Build history of the part. All positions in model axes, mm. Face numbers are marked on the shaded views. A direction names the side the tool comes from. Round coordinates to 2 decimals unless told otherwise and drop trailing zeros. Loops run counter-clockwise (first coordinate to the right, second up) from the corner with the lowest first, then second, coordinate; pieces in that order, holes last. Notation, with made-up numbers: (86.25, -1) - (109.25, -1) arc R18 cw to (109.25, 28) - close; hole circle Ø3 at (-1, 58). An arc over 180 degrees is marked (long way). Put each result on its own line as item: value. Start each with the question number.
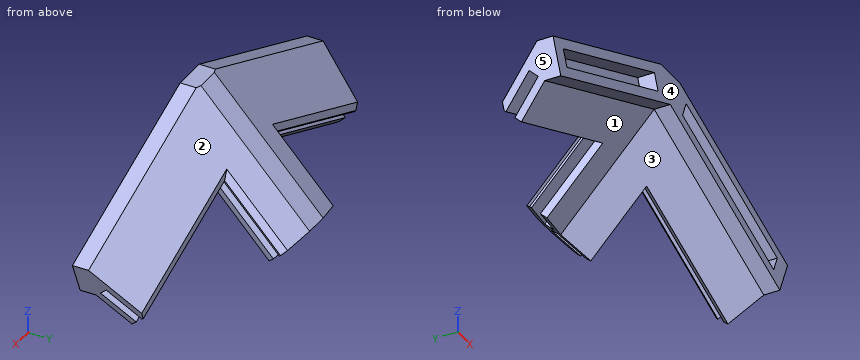
from build123d import *

# Parameters (mm, degrees)
SKETCH1_W                = 214.0895226738578
SKETCH1_H                = 271.0335668448457
BOSS_EXTRUDE1_DEPTH      = 10
SKETCH3_W                = 107.0447613369289
SKETCH3_H                = 271.0335668448457
CUT_EXTRUDE1_DEPTH       = 252.25359017903727
CUT_EXTRUDE2_DEPTH       = 249.55642867000518
BOSS_EXTRUDE3_DEPTH      = 40
CUT_EXTRUDE3_START       = -165.689856025
CUT_EXTRUDE3_DEPTH       = 205.862728092
CUT_EXTRUDE4_DEPTH       = 250.9605933606232
CUT_EXTRUDE5_DEPTH       = 250.96059336062322
BOSS_EXTRUDE5_DEPTH      = 45.000000000000014
CUT_EXTRUDE7_DEPTH       = 253.78419033582136
CUT_EXTRUDE9_DEPTH       = 253.78419033582136
CUT_EXTRUDE10_DEPTH      = 105
BOSS_EXTRUDE6_DEPTH      = 13.546139965279659
BOSS_EXTRUDE7_DEPTH      = 30
CUT_EXTRUDE12_DEPTH      = 30
CUT_EXTRUDE13_DEPTH      = 30
CUT_EXTRUDE14_DEPTH      = 30
CUT_EXTRUDE14_DEPTH_BACK = 101.66514829221025
BOSS_EXTRUDE8_DEPTH      = 5.2
CHAMFER1_START           = 223.359720619
CHAMFER1_OUTLINE_W       = 14
CHAMFER1_OUTLINE_H       = 9.000000000000002
CHAMFER1_DEPTH           = 3.640279381
CHAMFER3_START           = 159.35770891
CHAMFER3_OUTLINE_W       = 10
CHAMFER3_OUTLINE_H       = 51.999999999999986
CHAMFER3_DEPTH           = 1.64229109
CHAMFER4_SIZE            = 1.7


with BuildPart() as part:
    # Sketch1 → Boss-Extrude1 (new body)
    with BuildSketch(Plane(origin=(0, 0, 0), x_dir=(1, 0, 0), z_dir=(0, 1, 0))):
        with Locations((-3.148375333439077, -90.06211454589605)):
            Rectangle(SKETCH1_W, SKETCH1_H)
    extrude(amount=BOSS_EXTRUDE1_DEPTH)

    # Sketch3 → Cut-Extrude1 (cut, through all)
    with BuildSketch(Plane(origin=(0, 10, 0), x_dir=(1, 0, 0), z_dir=(0, 1, 0))):
        with Locations((-56.67075600190353, -90.06211454589605)):
            Rectangle(SKETCH3_W, SKETCH3_H)
    extrude(amount=-CUT_EXTRUDE1_DEPTH, mode=Mode.SUBTRACT)

    # Sketch4 → Cut-Extrude2 (cut, through all)
    with BuildSketch(Plane(origin=(0, 10, 0), x_dir=(1, 0, 0), z_dir=(0, 1, 0))):
        Polygon((103.89638600348982, -181.2395060415717), (100.8349185445691, -173.8484697814814), (9.99658424143476, 45.454668876526796), (103.89638600348982, 45.454668876526796), align=None)
    extrude(amount=-CUT_EXTRUDE2_DEPTH, mode=Mode.SUBTRACT)

    # Sketch6 → Boss-Extrude3 (add, along a direction that is not the sketch's normal)
    with BuildSketch(Plane(origin=(0, 10, 0), x_dir=(1, 0, 0), z_dir=(0, 1, 0))):
        Polygon((99.57206321776432, -170.7996673241942), (103.89638600348982, -181.2395060415717), (-3.148375333439077, -225.57889796831887), (-3.148375333439077, -213.34786610501484), align=None)
    extrude(amount=BOSS_EXTRUDE3_DEPTH, dir=(-0.2705980500730979, 0.7071067811865489, -0.6532814824381872))

    # Cut-Extrude3: read off the stored shape, not the designer's step
    # Cut-Extrude3 outline → Cut-Extrude3 (cut)
    with BuildSketch(Plane(origin=(0, 0, 0), x_dir=(1, 0, 0), z_dir=(0, 0.6785983445458481, -0.7345095552677544)).offset(CUT_EXTRUDE3_START)):
        Polygon((-3.148375333, -165), (-3.148375333, -152.122604304), (-13.972297336, -155.165042499), (-15, -155.45391393), (-15, -165), align=None)
    extrude(amount=CUT_EXTRUDE3_DEPTH, mode=Mode.SUBTRACT)

    # Sketch8 → Cut-Extrude4 (cut, through all)
    with BuildSketch(Plane(origin=(0, 10, 0), x_dir=(1, 0, 0), z_dir=(0, 1, 0))):
        Polygon((-3.1483753334390765, -225.5788979683189), (103.89638600348982, -181.2395060415717), (103.89638600348982, -225.57889796831887), align=None)
    extrude(amount=-CUT_EXTRUDE4_DEPTH, mode=Mode.SUBTRACT)

    # Sketch9 → Cut-Extrude5 (cut, through all)
    with BuildSketch(Plane(origin=(0, 10, 0), x_dir=(1, 0, 0), z_dir=(0, 1, 0))):
        Polygon((-3.1483753334390765, -213.34786610501484), (99.57206321776434, -170.7996673241942), (9.99658424143476, 45.454668876526796), (-3.148375333439077, 45.454668876526796), align=None)
    extrude(amount=-CUT_EXTRUDE5_DEPTH, mode=Mode.SUBTRACT)

    # Sketch13 → Boss-Extrude5 (add)
    with BuildSketch(Plane.XZ):
        Polygon((-3.1483753334390765, 225.5788979683189), (-3.1483753334390765, 213.34786610501484), (99.57206321776434, 170.7996673241942), (103.89638600348982, 181.23950604157167), align=None)
    extrude(amount=BOSS_EXTRUDE5_DEPTH)

    # Sketch14 → Cut-Extrude7 (cut, through all)
    with BuildSketch(Plane(origin=(24.60327067321852, 0, -10.191008391583336), x_dir=(-0.38268343236508967, 0, -0.9238795325112868), z_dir=(0.9238795325112867, 0, -0.3826834323650896))):
        Polygon((-178.9186244729457, 38.28427124746196), (-173.2686244729457, 32.63427124746195), (-167.6186244729457, 38.28427124746196), align=None)
    extrude(amount=-CUT_EXTRUDE7_DEPTH, mode=Mode.SUBTRACT)

    # Sketch21 → Cut-Extrude9 (cut, through all)
    with BuildSketch(Plane(origin=(24.60327067321852, 0, -10.191008391583336), x_dir=(-0.38268343236508967, 0, -0.9238795325112868), z_dir=(0.9238795325112867, 0, -0.3826834323650896))):
        Polygon((-178.9186244729457, 38.28427124746196), (-173.26862447294567, 32.63427124746195), (-186.71050756498246, 19.192388155425135), (-188.37220850077088, 20.854089091213513), (-197.564596656196, 11.661700935788378), (-199.8911947846192, 13.988299064211581), (-190.69880662919408, 23.180687219636717), (-192.3605075649825, 24.84238815542509), align=None)
    extrude(amount=-CUT_EXTRUDE9_DEPTH, mode=Mode.SUBTRACT)

    # Sketch26 → Cut-Extrude10 (cut)
    with BuildSketch(Plane(origin=(24.60327067321852, 0, -10.191008391583336), x_dir=(-0.38268343236508967, 0, -0.9238795325112868), z_dir=(0.9238795325112867, 0, -0.3826834323650896))):
        Polygon((-195.9028957204076, -45.000000000000014), (-207.2028957204075, -45.000000000000014), (-207.20289572040753, 4.999999999999999), (-204.20289572040753, 4.999999999999999), (-204.20289572040753, 10.2), (-198.9028957204076, 10.200000000000001), (-198.9028957204076, 5), (-195.9028957204076, 5), align=None)
    extrude(amount=-CUT_EXTRUDE10_DEPTH, mode=Mode.SUBTRACT)

    # Sketch27 → Boss-Extrude6 (add, along a direction that is not the sketch's normal)
    with BuildSketch(Plane(origin=(35.57097911044696, -92.95144786020374, 85.87594019533113), x_dir=(0.9626924198811571, 0.19875685341551327, -0.18362738881693624), z_dir=(-0.2705980500730966, 0.7071067811865525, -0.6532814824381838))):
        Polygon((-40.21986009681666, -165.94075499699434), (-39.260177114555994, -165.65967035927952), (-38.33532246822035, -168.81732163602243), (-40.219860096816646, -169.36928992803706), align=None)
    extrude(amount=BOSS_EXTRUDE6_DEPTH, dir=(0, 0.6785983445458494, -0.7345095552677533))

    # Sketch28 → Boss-Extrude7 (add, along a direction that is not the sketch's normal)
    with BuildSketch(Plane(origin=(32.05320445949652, -83.75905970477851, 77.38328092363429), x_dir=(0.9626924198811573, 0.1987568534155131, -0.18362738881693524), z_dir=(-0.27059805007309584, 0.7071067811865541, -0.6532814824381823))):
        Polygon((-23.13019805487444, -160.93530887309606), (-23.79074695350427, -158.6800538647835), (-36.56575980652385, -162.4217684996877), (-36.565759806523836, -170.74775403356227), (-21.544794509909032, -166.34821515815156), (-22.205343408538862, -164.09296014983897), (-34.68122217792752, -167.7470604401317), (-35.606076824263106, -164.58940916338878), align=None)
    extrude(amount=BOSS_EXTRUDE7_DEPTH, dir=(0, 0.6785983445458483, -0.7345095552677544))

    # Sketch29 → Cut-Extrude12 (cut)
    with BuildSketch(Plane(origin=(41.559974826961344, 108.60144786020382, 100.33465487913432), x_dir=(0.9626924198811563, -0.1987568534155138, -0.18362738881693985), z_dir=(0.2705980500730995, 0.7071067811865461, 0.6532814824381895))):
        Polygon((-46.44094960872295, -107.03174707988727), (-31.419984312108156, -107.03174707988727), (-31.41998431210815, -102.63220820447661), align=None)
    extrude(amount=-CUT_EXTRUDE12_DEPTH, mode=Mode.SUBTRACT)

    # Sketch30 → Cut-Extrude13 (cut)
    with BuildSketch(Plane(origin=(-72.40408024046648, 0, 29.990752006750984), x_dir=(-0.3826834323650857, 0, -0.9238795325112884), z_dir=(0.9238795325112884, 0, -0.3826834323650857))):
        Polygon((-207.20289572040787, 4.610357956966736), (-207.20289572040795, -45.000000000000014), (-195.90289572040788, -45.000000000000014), (-195.90289572040788, 4.6103579569667374), (-195.9028957204076, 5), (-207.20289572040755, 4.999999999999999), align=None)
    extrude(amount=-CUT_EXTRUDE13_DEPTH, mode=Mode.SUBTRACT)

    # Sketch31 → Cut-Extrude14 (cut, two sides: drawn at the far end of the back side and taken through both)
    with BuildSketch(Plane(origin=(74.968792544546, 0, 180.99067571577757), x_dir=(-0.9238795325112865, 0, 0.38268343236509056), z_dir=(-0.38268343236509056, 0, -0.9238795325112865)).offset(-CUT_EXTRUDE14_DEPTH_BACK)):
        Polygon((18.0534132200626, -1.4270293234233122), (-26.630388278374163, -1.4270293234233173), (-26.630388278374163, 30.311404517874507), (18.0534132200626, 30.311404517874507), align=None)
    extrude(amount=CUT_EXTRUDE14_DEPTH + CUT_EXTRUDE14_DEPTH_BACK, mode=Mode.SUBTRACT)

    # Sketch33 → Boss-Extrude8 (add)
    with BuildSketch(Plane(origin=(1.28e-15, 10.200000000000065, 3.08e-15), x_dir=(-1, 1.3e-16, 0), z_dir=(-1.3e-16, -1, -3e-16))):
        Polygon((-61.46588606719166, -195.56761797257994), (-56.84648840463523, -197.48103513440537), (-54.81826621310026, -192.5844736120956), (-59.437663875656696, -190.67105645027016), align=None)
    extrude(amount=BOSS_EXTRUDE8_DEPTH)

    # Mirror4: part across plane


with BuildPart() as part_1:
    add(part.part)
    add(part.part.mirror(Plane(origin=(-3.148375333439077, 0, 225.57889796831887), x_dir=(0, 0, 1), z_dir=(1, 0, 0))))

    # Chamfer1: read off the stored shape, not the designer's step
    # Chamfer1 outline → Chamfer1 (cut)
    with BuildSketch(Plane.XY.offset(CHAMFER1_START)):
        with Locations((-3, 9.5)):
            Rectangle(CHAMFER1_OUTLINE_W, CHAMFER1_OUTLINE_H)
    extrude(amount=CHAMFER1_DEPTH, mode=Mode.SUBTRACT)

    # Chamfer3: read off the stored shape, not the designer's step
    # Chamfer3 outline → Chamfer3 (cut)
    with BuildSketch(Plane(origin=(0, 0, 0), x_dir=(1, 0, 0), z_dir=(0, 0.7345095552677543, 0.6785983445458483)).offset(CHAMFER3_START)):
        with Locations((-3, -132)):
            Rectangle(CHAMFER3_OUTLINE_W, CHAMFER3_OUTLINE_H)
    extrude(amount=CHAMFER3_DEPTH, mode=Mode.SUBTRACT)

    # Chamfer4
    chamfer4_edges = [part_1.edges().sort_by_distance(p)[0] for p in [
        (34.12309720869192, 24.84238815542509, 194.07526337860742),
        (11.312194096909927, 33.52860342480338, 194.1219571598504),
        (-17.60894476378808, 33.52860342480338, 194.1219571598504),
        (-40.41984787557007, 24.84238815542509, 194.07526337860742),
    ]]
    chamfer(chamfer4_edges, length=CHAMFER4_SIZE)


solid = part_1.part
1) Drop flat-ended pins along their axis: pin 1 Ø6.5 at (x, z) = (-49.5, 190) entering from +Y; pin 2 Ø8 at (x, y) = (-33, 26.5) entering from -Z; pin 3 Ø3 at (x, y) = (5.5, 36) entering from -Z. Give the stop position or say it passes through.
2) Pull direction X, two halves, no side cores. Call the marked faces 3, 4 and 5: pulls with the +X half, pulls with the -X half, needs draft (parallel to the pull), parting line crosses it, or undercut.
3) Slice it at B-B, the plane x = 46.5. Write the cut outline in (y, z), and give its area (3 significant figures).
4) Slice it at A-A, the plane z = 208. Write the cut outline in (x, y).
5) Drill centre lines: line 1 (Z direction, x = -46, y = 19.5); line 2 (Z direction, x = -1, y = 36); line 3 (Y direction, x = 27, z = 205). Where is each one in solid material? Low to high. Write a range as [from, to].
6) Which spindle directions (+Z, -Z, +X, -X, +Y, -Y) get a long thin tool onto all of the face, cutting with end or side? Do the marked faces 1 and 2. Say none if no direction does.
7) Slice it at C-C, the plane z = 194. State how many separate pieces and enclosed holes the cut face has, and give its area (3 significant figures).
8) Slice it at D-D, the plane y = 30. Write the cut outline in (x, z).
Taken from the geometry:
1. pin 1: stops at y = 23.64
1. pin 2: stops at z = 194.43
1. pin 3: stops at z = 180
2. face 3: undercut
2. face 4: needs draft
2. face 5: pulls with the -X half
3. outline: (5, 192.78) - (10, 192.78) - (19.19, 182.83) - (20.85, 184.63) - (11.66, 194.58) - (13.99, 197.1) - (23.18, 187.15) - (23.64, 187.65) - (23.64, 190.25) - (10, 205.01) - (5, 205.01) - (5, 201.77) - (10.2, 201.77) - (10.2, 196.03) - (5, 196.03) - close
3. area: 130 mm2
4. outline: (-45.59, 5) - (-37.75, 5) - (-37.75, 10.2) - (-23.9, 10.2) - (-23.9, 5) - (-16.06, 5) - (-16.06, 10) - (-3.15, 14.94) - (9.76, 10) - (9.76, 5) - (17.6, 5) - (17.6, 10.2) - (31.45, 10.2) - (31.45, 5) - (39.29, 5) - (39.29, 10) - (0.64, 24.79) - (-6.94, 24.79) - (-45.59, 10) - close; hole (-26.48, 13.99) - (-20.4, 11.66) - (-4.07, 17.91) - (-4.96, 22.22) - close; hole (-2.22, 17.91) - (14.1, 11.66) - (20.18, 13.99) - (-1.33, 22.22) - close
5. line 1: z = [185.98, 188.91], [193.95, 197.55]
5. line 2: z = [184.32, 187.91], [192.95, 195.87]
5. line 3: y = [10.2, 13.82], [14.15, 17.48]
6. face 1: -Z, -Y
6. face 2: +Z, +X, +Y
7. separate pieces: 3
7. enclosed holes: 0
7. area: 733 mm2
8. outline: (-17.15, 195.53) - (-16.97, 194.61) - (-4.96, 199.58) - (-4.07, 194.91) - (-16.08, 189.94) - (-15.45, 186.61) - (-3.15, 191.7) - (9.15, 186.61) - (9.79, 189.94) - (-2.22, 194.91) - (-1.33, 199.58) - (10.68, 194.61) - (10.85, 195.53) - (9.68, 198.62) - (0.64, 202.36) - (-6.94, 202.36) - (-15.97, 198.62) - close
